Verification items for the finished model (mm, model axes). A direction names the side the tool comes from. Round coordinates to 2 decimals unless told otherwise and drop trailing zeros. Loops run counter-clockwise (first coordinate to the right, second up) from the corner with the lowest first, then second, coordinate; pieces in that order, holes last. Notation, with made-up numbers: (-31.75, -24) -> (-14.75, -24) arc R7 cw to (-14.75, -18) -> close; hole circle Ø10 at (3, -21). An arc over 180 degrees is marked (long way). Write item = value, one per line. Start each with the question number.
```python
from build123d import *

# Parameters (mm, degrees)
BOSS_EXTRUDE1_DEPTH   = 40
BODY_MOVE_COPY1_ANGLE = 20
BOSS_EXTRUDE2_DEPTH   = 2
SKETCH1_4_W           = 81
SKETCH1_4_H           = 35
BOSS_EXTRUDE3_DEPTH   = 12
SKETCH4_R             = 2.5
CUT_EXTRUDE2_DEPTH    = 8
FILLET1_R             = 2
SKETCH10_W            = 4.9
SKETCH10_H            = 3
SKETCH10_W_2          = 5.1
SKETCH10_W_3          = 5
CUT_EXTRUDE4_DEPTH    = 2
FILLET2_R             = 0.5


with BuildPart() as part:
    # Sketch2 → Boss-Extrude1 (new body)
    with BuildSketch(Plane.XY):
        Polygon((90, 0), (102, 0), (102, 2), (92, 25), (90, 25), align=None)
    extrude(amount=BOSS_EXTRUDE1_DEPTH)


with BuildPart() as part_1:
    # Body-Move/Copy1: moved
    add(part.part.rotate(Axis((95, 0, 20), (0, -1, 0)), BODY_MOVE_COPY1_ANGLE))


with BuildPart() as part_2:
    # Body-Move/Copy2: moved
    add(part_1.part.moved(Location((-4, 0, -25))))

    # Sketch1 → Boss-Extrude2 (add)
    with BuildSketch(Plane(origin=(0, 0, 0), x_dir=(1, 0, 0), z_dir=(0, 1, 0))):
        Polygon((0, 0), (73, 0), (84, -12), (87, 0), (87, 87), (0, 87), align=None)
    extrude(amount=BOSS_EXTRUDE2_DEPTH)

    # Sketch1<4> → Boss-Extrude3 (add)
    with BuildSketch(Plane(origin=(0, 0, 0), x_dir=(1, 0, 0), z_dir=(0, 1, 0))):
        Polygon((8, 43), (8, 46), (39.9, 46), (39.9, 43), (44.9, 43), (44.9, 46), (79, 46), (79, 43), (83.9, 43), (83.9, 6), (79, 6), (79, 3), (44.9, 3), (44.9, 6), (39.9, 6), (39.9, 3), (8, 3), (8, 6), (2.9, 6), (2.9, 13), (0, 13), (0, 0), (87, 0), (87, 87), (0, 87), (0, 36), (2.9, 36), (2.9, 43), align=None)
        with Locations((43.5, 66.5)):
            Rectangle(SKETCH1_4_W, SKETCH1_4_H, mode=Mode.SUBTRACT)
    extrude(amount=BOSS_EXTRUDE3_DEPTH)

    # Sketch4 → Cut-Extrude2 (cut)
    with BuildSketch(Plane(origin=(72.447790922, 33.520577724, 26.368839434), x_dir=(0.30020671045987535, 0.09758957417323016, -0.948868908757974), z_dir=(0.8617639646050662, 0.3987261114144503, 0.31365643207890637))):
        with Locations(Location((42.044187921, -18.952687866, 0), (0, 0, 92.148700458))):
            Circle(SKETCH4_R)
        with Locations(Location((40.341555526, -34.861837527, 0), (0, 0, 92.148700458))):
            Circle(SKETCH4_R)
    extrude(amount=-CUT_EXTRUDE2_DEPTH, mode=Mode.SUBTRACT)

    # Fillet1
    fillet1_edges = [part_2.edges().sort_by_distance(p)[0] for p in [
        (80.40082665, 25, 12.425771842),
        (94.081632383, 25, -25.161932989),
    ]]
    fillet(fillet1_edges, radius=FILLET1_R)

    # Sketch10 → Cut-Extrude4 (cut)
    with BuildSketch(Plane(origin=(0, 12, 0), x_dir=(1, 0, 0), z_dir=(0, 1, 0))):
        with Locations((81.45, 4.5)):
            Rectangle(SKETCH10_W, SKETCH10_H)
        with Locations((42.45, 4.5)):
            Rectangle(SKETCH10_W_2, SKETCH10_H)
        with Locations((42.4, 44.5)):
            Rectangle(SKETCH10_W_3, SKETCH10_H)
        with Locations((81.45, 44.5)):
            Rectangle(SKETCH10_W, SKETCH10_H)
        with Locations((5.45, 44.5)):
            Rectangle(SKETCH10_W_2, SKETCH10_H)
        with Locations((5.45, 4.5)):
            Rectangle(SKETCH10_W_2, SKETCH10_H)
    extrude(amount=-CUT_EXTRUDE4_DEPTH, mode=Mode.SUBTRACT)

    # Fillet2
    fillet2_edges = [part_2.edges().sort_by_distance(p)[0] for p in [
        (43.4, 12, -3),
        (43.5, 12, -49),
        (86.301536896, 25, -6.710100717),
        (79.46113403, 11.5, 12.083751699),
        (93.141939763, 11.5, -25.503953132),
        (79.661484791, 24.414213562, 11.533292506),
        (92.941589001, 24.414213562, -24.95349394),
        (87, 6, -87),
        (0, 6, -87),
        (0, 6, 0),
        (3, 12, -66.5),
        (43.5, 12, -84),
        (84, 12, -66.5),
        (2.9, 12, -41),
        (43.4, 12, -46),
        (83.9, 12, -24.5),
        (2.9, 12, -8),
    ]]
    fillet(fillet2_edges, radius=FILLET2_R)


solid = part_2.part
```
(1) Section check C-C on z = -32.5. Enter the section's corners in (x, y), then the cut area to 3 significant figures.
(2) Access from +Z, -Z, +X, -X, +Y, -Y to the whole of each face (thin tool, end or side, straight path). Record for faces 1 (the cylindrical face through (86.35, 24.85, -6.42)), 2 (the flat face through (81, 6, -43)), 3 (the flat face through (80, 2, 3)).
(3) Scan lines: line 1 (Z direction, x = 16, y = 11.5); line 2 (Y direction, x = 27.5, z = -18.5); line 3 (X direction, y = 9.75, z = -66). Record each from-to range of solid material in increasing order. Write a range as [from, to].
(4) Section check B-B on z = -74.5. Enter the section's corners in (x, y).
(5) Section check A-A on x = 30. Enter the section's corners in (y, z).
(6) Depth check by flat-ended pin: pin 1 Ø1 at (x, z) = (57.5, -43) entering from +Y; pin 2 Ø3.5 at (y, z) = (4, -45) entering from +X; pin 3 Ø2.5 at (x, z) = (82, -4.5) entering from +Y; pin 4 Ø10.5 at (y, z) = (4.5, -29) entering from -X. Enter the tip coordinate at first touch or a pass-through.
(7) Draft check along Y on faces 4 (the flat face through (88, 25, -7)), 5 (the cylindrical face through (94.2, 6.16, -11.19)), 6 (the flat face through (51, 0, -36)), 7 (the flat face through (3, 7, -66)). Enter one of: +Y half, -Y half, draft (parallel to the pull), parting line (faces both ways), or undercut.
Computed values:
q1.outline = (0, 0) -> (87, 0) -> (87, 12) -> (84.4, 12) arc R0.5 ccw to (83.9, 11.5) -> (83.9, 2) -> (0, 2) -> close
q1.area = 205 mm²
q2.face_1 = -Z, -X, +Y
q2.face_2 = +Y
q2.face_3 = -X, +Y
q3.line_1 = [-87, -84], [-49, -46], [-3, 0]
q3.line_2 = [0, 2]
q3.line_3 = [0, 3], [84, 87]
q4.outline = (0, 0) -> (87, 0) -> (87, 12) -> (84.5, 12) arc R0.5 ccw to (84, 11.5) -> (84, 2) -> (3, 2) -> (3, 11.5) arc R0.5 ccw to (2.5, 12) -> (0, 12) -> close
q5.outline = (0, -87) -> (12, -87) -> (12, -84.5) arc R0.5 ccw to (11.5, -84) -> (2, -84) -> (2, -49) -> (11.5, -49) arc R0.5 ccw to (12, -48.5) -> (12, -46.5) arc R0.5 ccw to (11.5, -46) -> (2, -46) -> (2, -3) -> (11.5, -3) arc R0.5 ccw to (12, -2.5) -> (12, 0) -> (0, 0) -> close
q6.pin_1 = 2
q6.pin_2 = 87
q6.pin_3 = 10
q6.pin_4 = 0
q7.face_4 = +Y half
q7.face_5 = undercut
q7.face_6 = -Y half
q7.face_7 = draft
